Read the model definition and answer for the solid it produces. Units are mm, in the model's axes. A direction names the side the tool comes from. Coordinates: 2 decimals unless noted, no trailing zeros. Loops run counter-clockwise (first coordinate to the right, second up) from the corner with the lowest first, then second, coordinate; pieces in that order, holes last. Notation, with made-up numbers: (7.5, 66.5) - (59.5, 66.5) arc R5 ccw to (59.5, 71.5) - close; hole circle Ø8 at (76.25, 5). An arc over 180 degrees is marked (long way). One line per item, written item: value. Start each with the question number.
from build123d import *

# Parameters (mm, degrees)
F1_DEPTH = 4
F2_W     = 5
F2_H     = 2.25
F2_W_2   = 8.75
F2_H_2   = 15
F2_H_3   = 21.6
F2_H_4   = 5
F3_DEPTH = 2
F4_DEPTH = 1


with BuildPart() as f1:
    # F0 (on Top) → F1 (new body)
    with BuildSketch(Plane.XY):
        with BuildLine():
            Line((48.6, 0), (3, 0))
            Line((3, 0), (3, -1.5))
            ThreePointArc((3, -1.5), (4.06066, -1.93934), (4.5, -3))
            ThreePointArc((4.5, -3), (3, -4.5), (1.5, -3))
            Line((1.5, -3), (0, -3))
            Line((0, -3), (0, -48.6))
            Line((0, -48.6), (1.5, -48.6))
            ThreePointArc((1.5, -48.6), (3, -47.1), (4.5, -48.6))
            ThreePointArc((4.5, -48.6), (4.06066, -49.66066), (3, -50.1))
            Line((3, -50.1), (3, -51.6))
            Line((3, -51.6), (48.6, -51.6))
            Line((48.6, -51.6), (48.6, -50.1))
            ThreePointArc((48.6, -50.1), (47.53934, -47.53934), (50.1, -48.6))
            Line((50.1, -48.6), (51.6, -48.6))
            Line((51.6, -48.6), (51.6, -3))
            Line((51.6, -3), (50.1, -3))
            ThreePointArc((50.1, -3), (47.53934, -4.06066), (48.6, -1.5))
            Line((48.6, -1.5), (48.6, 0))
        make_face()
        with BuildLine():
            Line((1.5, -48.6), (0, -48.6))
            Line((0, -48.6), (0, -51.6))
            Line((0, -51.6), (3, -51.6))
            Line((3, -51.6), (3, -50.1))
            ThreePointArc((3, -50.1), (1.93934, -49.66066), (1.5, -48.6))
        make_face()
        with BuildLine():
            Line((51.6, -51.6), (51.6, -48.6))
            Line((51.6, -48.6), (50.1, -48.6))
            ThreePointArc((50.1, -48.6), (49.66066, -49.66066), (48.6, -50.1))
            Line((48.6, -50.1), (48.6, -51.6))
            Line((48.6, -51.6), (51.6, -51.6))
        make_face()
        with BuildLine():
            Line((51.6, 0), (48.6, 0))
            Line((48.6, 0), (48.6, -1.5))
            ThreePointArc((48.6, -1.5), (49.66066, -1.93934), (50.1, -3))
            Line((50.1, -3), (51.6, -3))
            Line((51.6, -3), (51.6, 0))
        make_face()
        with BuildLine():
            Line((3, 0), (0, 0))
            Line((0, 0), (0, -3))
            Line((0, -3), (1.5, -3))
            ThreePointArc((1.5, -3), (1.93934, -1.93934), (3, -1.5))
            Line((3, -1.5), (3, 0))
        make_face()
    extrude(amount=F1_DEPTH)

    # F2 (on face) → F3 (cut)
    with BuildSketch(Plane.XY.offset(4)):
        with Locations((3.75, -9.875)):
            Rectangle(F2_W, F2_H)
        with Locations((4.375, -27)):
            Rectangle(F2_W_2, F2_H_2)
        with BuildLine():
            Line((16, -37.6), (13.7, -37.6))
            ThreePointArc((13.7, -37.6), (14.373654, -39.226346), (16, -39.9))
            Line((16, -39.9), (16, -37.6))
        make_face()
        with BuildLine():
            ThreePointArc((18.3, -37.6), (16, -35.3), (13.7, -37.6))
            Line((13.7, -37.6), (16, -37.6))
            Line((16, -37.6), (16, -39.9))
            ThreePointArc((16, -39.9), (17.626346, -39.226346), (18.3, -37.6))
        make_face()
        with BuildLine():
            ThreePointArc((37.9, -37.6), (33.973654, -35.973654), (35.6, -39.9))
            Line((35.6, -39.9), (35.6, -37.6))
            Line((35.6, -37.6), (37.9, -37.6))
        make_face()
        with BuildLine():
            Line((35.6, -37.6), (35.6, -39.9))
            ThreePointArc((35.6, -39.9), (37.226346, -39.226346), (37.9, -37.6))
            Line((37.9, -37.6), (35.6, -37.6))
        make_face()
        with Locations((47.225, -26.8)):
            Rectangle(F2_W_2, F2_H_3)
        with Locations((47.225, -40.1)):
            Rectangle(F2_W_2, F2_H_4)
        with Locations((10, -3.025)):
            Rectangle(F2_W, F2_H)
    extrude(amount=-F3_DEPTH, mode=Mode.SUBTRACT)

    # F2 (on face) → F4 (cut)
    with BuildSketch(Plane.XY.offset(4)):
        with BuildLine():
            Line((13.7, -37.6), (0, -37.6))
            Line((0, -37.6), (0, -45.6))
            Line((0, -45.6), (6, -45.6))
            Line((6, -45.6), (6, -51.6))
            Line((6, -51.6), (16, -51.6))
            Line((16, -51.6), (16, -39.9))
            ThreePointArc((16, -39.9), (14.373654, -39.226346), (13.7, -37.6))
        make_face()
        with BuildLine():
            Line((6, -6), (0, -6))
            Line((0, -6), (0, -19.5))
            Line((0, -19.5), (8.75, -19.5))
            Line((8.75, -19.5), (8.75, -34.5))
            Line((8.75, -34.5), (0, -34.5))
            Line((0, -34.5), (0, -37.6))
            Line((0, -37.6), (13.7, -37.6))
            ThreePointArc((13.7, -37.6), (16, -35.3), (18.3, -37.6))
            ThreePointArc((18.3, -37.6), (17.626346, -39.226346), (16, -39.9))
            Line((16, -39.9), (16, -51.6))
            Line((16, -51.6), (35.6, -51.6))
            Line((35.6, -51.6), (35.6, -39.9))
            ThreePointArc((35.6, -39.9), (33.973654, -35.973654), (37.9, -37.6))
            Line((37.9, -37.6), (42.85, -37.6))
            Line((42.85, -37.6), (42.85, -16))
            Line((42.85, -16), (51.6, -16))
            Line((51.6, -16), (51.6, -6))
            Line((51.6, -6), (45.6, -6))
            Line((45.6, -6), (45.6, 0))
            Line((45.6, 0), (6, 0))
            Line((6, 0), (6, -6))
        make_face()
        with Locations((3.75, -9.875)):
            Rectangle(F2_W, F2_H, mode=Mode.SUBTRACT)
        with Locations((10, -3.025)):
            Rectangle(F2_W, F2_H, mode=Mode.SUBTRACT)
        with BuildLine():
            Line((35.6, -39.9), (35.6, -51.6))
            Line((35.6, -51.6), (45.6, -51.6))
            Line((45.6, -51.6), (45.6, -45.6))
            Line((45.6, -45.6), (51.6, -45.6))
            Line((51.6, -45.6), (51.6, -42.6))
            Line((51.6, -42.6), (42.85, -42.6))
            Line((42.85, -42.6), (42.85, -37.6))
            Line((42.85, -37.6), (37.9, -37.6))
            ThreePointArc((37.9, -37.6), (37.226346, -39.226346), (35.6, -39.9))
        make_face()
    extrude(amount=-F4_DEPTH, mode=Mode.SUBTRACT)


solid = f1.part
1) Section C-C, the plane y = -41 is taken. Determine the outline of the cut face in (x, z), and give its area (3 significant figures).
2) Section B-B, the plane x = 22.5 is taken. Determine the outline of the cut face in (y, z).
3) Straight lines are drawn through the part: L1, parallel to X at y = -48.6, z = 1.45; L2, parallel to X at y = -3, z = 2.4; L3, parallel to Y at x = 48.6, z = 3.2. For each, find the intervals that lie inside material, in ascending order.
4) For faces 4 (the flat face through (47, -29, 2)), 5 (the flat face through (4, -27, 2)), 6 (the flat face through (25, -51.6, 2)), 7 (the flat face through (16, -38, 2)), 8 (the flat face through (1.6, -1.6, 4)), determine the directions among +Z, -Z, +X, -X, +Y, -Y from which every point of the face is accessible in a straight line to the end or side of a thin tool.
5) Section A-A, the plane y = -26.5 is taken. Determine the outline of the cut face in (x, z), and give its area (3 significant figures).
6) Flat-ended cylindrical pins translate along their axes: P1, Ø1.8, axis at x = 48.6, y = -48.6, coming from the -Z side; P2, Ø8, axis at x = 42.5, y = -20.5, coming from the +Z side; P3, Ø1.1, axis at x = 4.5, y = -10, coming from the +Z side. Find the tip coordinate at first contact, or state that the pin passes through.
7) Determine the mould class of faces 1 (the flat face through (26, 0, 2)), 2 (the flat face through (51.6, -26.2, 1.5)), 3 (the flat face through (25, -25, 3)) for opening direction X: released by +X, released by -X, zero draft, split by the parting line, or undercut.
Answer below:
1. outline: (0, 0) - (51.6, 0) - (51.6, 2) - (42.85, 2) - (42.85, 3) - (0, 3) - close
1. area: 146 mm2
2. outline: (-51.6, 0) - (0, 0) - (0, 3) - (-51.6, 3) - close
3. L1: 0 to 1.5, 4.5 to 47.1, 50.1 to 51.6
3. L2: 0 to 1.5, 4.5 to 7.5, 12.5 to 47.1, 50.1 to 51.6
3. L3: -51.6 to -50.1, -47.1 to -45.6, -6 to -4.5, -1.5 to 0
4. face 4: +Z, +X
4. face 5: +Z, -X
4. face 6: +Z, -Z, +X, -X, -Y
4. face 7: +Z
4. face 8: +Z, +X, -X, +Y, -Y
5. outline: (0, 0) - (51.6, 0) - (51.6, 2) - (42.85, 2) - (42.85, 3) - (8.75, 3) - (8.75, 2) - (0, 2) - close
5. area: 137 mm2
6. P1: through
6. P2: z = 3
6. P3: z = 2
7. face 1: zero draft
7. face 2: released by +X
7. face 3: undercut
